Autodesk Fusion 360 part; units mm, degrees
sketch "Sketch1" plane through (0, 0, 0) normal (0, 0, 1) x (1, 0, 0)
  line L0 (-77.1661, 21.8494) -> (-77.196, -36.9915)
  line L1 (-55.1143, 21.8382) -> (-77.1661, 21.8494)
  line L2 (-55.1022, 45.5931) -> (-55.1143, 21.8382)
  line L3 (-35.4199, 45.5831) -> (-55.1022, 45.5931)
  line L4 (-35.4199, 55.6506) -> (-35.4199, 45.5831)
  line L5 (-16.3374, 55.6581) -> (-35.4199, 55.6506)
  line L6 (-16.3374, 65.0231) -> (-16.3374, 55.6581)
  line L7 (5.0551, 65.0106) -> (-16.3374, 65.0231)
  line L8 (5.0551, 55.3606) -> (5.0551, 65.0106)
  line L9 (24.2287, 55.413) -> (5.0551, 55.3606)
  line L10 (24.2287, 45.8698) -> (24.2287, 55.413)
  line L11 (43.6774, 45.8599) -> (24.2287, 45.8698)
  line L12 (43.6724, 36.0748) -> (43.6774, 45.8599)
  line L13 (72.4097, 36.0602) -> (43.6724, 36.0748)
  line L14 (72.377, -28.4302) -> (72.4097, 36.0602)
  line L15 (-18.082, -28.4553) -> (72.377, -28.4302)
  line L16 (-18.0799, -36.9775) -> (-18.082, -28.4553)
  line L17 (-77.196, -36.9915) -> (-18.0799, -36.9775)
  line L18 (-18.8374, 67.5106) -> (7.5551, 67.5106)
  line L19 (7.5551, 67.5106) -> (7.5551, 57.913)
  line L20 (7.5551, 57.913) -> (26.7287, 57.913)
  line L21 (26.7287, 57.913) -> (26.7287, 48.3599)
  line L22 (26.7287, 48.3599) -> (46.1774, 48.3599)
  line L23 (46.1774, 48.3599) -> (46.1774, 38.5602)
  line L24 (74.9097, 38.5602) -> (46.1774, 38.5602)
  line L25 (74.9097, 38.5602) -> (74.8744, -30.9302)
  line L26 (-15.5799, -30.9553) -> (-15.5799, -39.4775)
  line L27 (-15.5799, -30.9553) -> (74.8744, -30.9302)
  line L28 (-15.5799, -39.4775) -> (-79.696, -39.4775)
  line L29 (-79.696, -39.4775) -> (-79.6636, 24.3382)
  line L30 (-79.6636, 24.3382) -> (-57.6022, 24.3382)
  line L31 (-57.6022, 24.3382) -> (-57.6022, 48.0931)
  line L32 (-57.6022, 48.0931) -> (-37.9199, 48.0931)
  line L33 (-37.9199, 58.1581) -> (-37.9199, 48.0931)
  line L34 (-37.9199, 58.1581) -> (-18.8374, 58.1581)
  line L35 (-18.8374, 58.1581) -> (-18.8374, 67.5106)
  dimension "d1" = 2.5
  dimension "d2" = 2.5
  dimension "d4" = 2.5
  dimension "d5" = 2.5
  dimension "d6" = 2.5
  dimension "d7" = 2.5
  dimension "d8" = 2.5
  dimension "d9" = 2.5
  dimension "d11" = 2.5
  dimension "d12" = 2.5
  dimension "d13" = 2.5
  dimension "d14" = 2.5
  dimension "d16" = 2.5
  dimension "d17" = 2.5
  dimension "d18" = 2.5
  dimension "d19" = 2.5
  dimension "d20" = 2.5
  dimension "d21" = 2.5
  dimension "d22" = 2.5
extrude "Extrude1" add sketch "Sketch1" along normal blind 13
extrude "Extrude2" add sketch "Sketch1" along normal blind 3 contours L0 L1 L2 L3 L4 L5 L6 L7 L8 L9 L10 L11 L12 L13 L14 L15 L16 L17
sketch "Sketch4" plane through (0, 0, 13) normal (0, 0, 1) x (-1, 0, 0)
  line L0 (18.0799, 36.9775) -> (77.196, 36.9915)
  line L1 (77.196, 36.9915) -> (77.1661, -21.8494)
  line L2 (77.1661, -21.8494) -> (55.1143, -21.8382)
  line L3 (55.1143, -21.8382) -> (55.1022, -45.5931)
  line L4 (55.1022, -45.5931) -> (35.4199, -45.5831)
  line L5 (35.4199, -45.5831) -> (35.4199, -55.6506)
  line L6 (35.4199, -55.6506) -> (16.3374, -55.6581)
  line L7 (16.3374, -55.6581) -> (16.3374, -65.0231)
  line L8 (16.3374, -65.0231) -> (-5.0551, -65.0106)
  line L9 (-5.0551, -65.0106) -> (-5.0551, -55.3606)
  line L10 (-5.0551, -55.3606) -> (-24.2287, -55.413)
  line L11 (-24.2287, -55.413) -> (-24.2287, -45.8698)
  line L12 (-24.2287, -45.8698) -> (-43.6774, -45.8599)
  line L13 (-43.6774, -45.8599) -> (-43.6724, -36.0748)
  line L14 (-43.6724, -36.0748) -> (-72.4097, -36.0602)
  line L15 (-72.4097, -36.0602) -> (-72.377, 28.4302)
  line L16 (-72.377, 28.4302) -> (18.082, 28.4553)
  line L17 (18.082, 28.4553) -> (18.0799, 36.9775)
  line L18 (37.9199, -58.1581) -> (37.9199, -48.0931)
  line L19 (37.9199, -48.0931) -> (57.6022, -48.0931)
  line L20 (57.6022, -48.0931) -> (57.6022, -24.3382)
  line L21 (57.6022, -24.3382) -> (79.6636, -24.3382)
  line L22 (79.6636, -24.3382) -> (79.696, 39.4775)
  line L23 (79.696, 39.4775) -> (15.5799, 39.4775)
  line L24 (15.5799, 39.4775) -> (15.5799, 30.9553)
  line L25 (15.5799, 30.9553) -> (-74.8744, 30.9302)
  line L26 (-74.8744, 30.9302) -> (-74.9097, -38.5602)
  line L27 (-74.9097, -38.5602) -> (-46.1774, -38.5602)
  line L28 (-46.1774, -38.5602) -> (-46.1774, -48.3599)
  line L29 (-46.1774, -48.3599) -> (-26.7287, -48.3599)
  line L30 (-26.7287, -48.3599) -> (-26.7287, -57.913)
  line L31 (-26.7287, -57.913) -> (-7.5551, -57.913)
  line L32 (-7.5551, -57.913) -> (-7.5551, -67.5106)
  line L33 (-7.5551, -67.5106) -> (18.8374, -67.5106)
  line L34 (18.8374, -67.5106) -> (18.8374, -58.1581)
  line L35 (18.8374, -58.1581) -> (37.9199, -58.1581)
  line L36 (73.8436, -24.8) -> (60.8436, -24.8)
  line L37 (60.8436, -24.8) -> (60.8436, -21.5)
  line L38 (60.8436, -21.5) -> (73.8436, -21.5)
  line L39 (73.8436, -21.5) -> (73.8436, -24.8)
  dimension "d27" = 13
  dimension "d28" = 5.82
extrude "Extrude3" cut sketch "Sketch4" against normal blind 6 contours L2 L21 L37 L39
fillet "Fillet1" radius 1 18 edges at (-79.696, -39.4775, 6.5) (-15.5799, -39.4775, 6.5) (-15.5799, -30.9553, 6.5) (74.8744, -30.9302, 6.5) (74.9097, 38.5602, 6.5) (46.1774, 38.5602, 6.5) (26.7287, 48.3599, 6.5) (46.1774, 48.3599, 6.5) (26.7287, 57.913, 6.5) (7.5551, 67.5106, 6.5) (7.5551, 57.913, 6.5) (-57.6022, 48.0931, 6.5) (-57.6022, 24.3382, 6.5) (-79.6636, 24.3382, 6.5) (-37.9199, 48.0931, 6.5) (-37.9199, 58.1581, 6.5) (-18.8374, 58.1581, 6.5) (-18.8374, 67.5106, 6.5)
Check sheet for the modelled part. Datum: model origin and axes. Units: mm. A direction names the side the tool comes from. Coordinates: 2 decimals unless noted, no trailing zeros. Order: outer loops, then holes, each group sorted by start corner. A loop starts at its lowest first (then second) coordinate and runs counter-clockwise, first axis right, second up. Notation, with made-up numbers: (8.25, 42) -> (55.25, 42) arc R10 cw to (55.25, 49) -> close; hole circle Ø1 at (46.5, 3.25). An arc over 180 degrees is marked (long way). Write item = value, one per line. Start each with the question number.
1) Mould release check, pull along Y, two halves, no side actions. Record for faces 1 (the flat face through (-47, -39.478, 6)), 2 (the flat face through (-3, 3, 3)), 3 (the flat face through (7.555, 63, 6)), 4 (the flat face through (-6, 67.511, 6)): +Y half, -Y half, draft (parallel to the pull), parting line (faces both ways), or undercut.
2) Go/stop test with flat-tipped pins: P1, Ø1, axis at y = 8.5, z = 3, coming from the +X side; P2, Ø6.5, axis at x = -47, z = 9, coming from the +Y side; P3, Ø3, axis at y = 51.5, z = 7.5, coming from the -X side. Record where each tip stops, or that it passes through.
3) Cross-section at B-B (y = 31.5). Enter the section's corners in (x, z).
4) Cross-section at A-A (x = -67). Enter the section's corners in (y, z).
5) Access from +Z, -Z, +X, -X, +Y, -Y to the whole of each face (thin tool, end or side, straight path). Record for faces 5 (the flat face through (-14, -29, 13)), 6 (the flat face through (-48, 48.093, 6)), 7 (the flat face through (36, 48.36, 6)).
6) Material ranges on L1, parallel to Y at x = 62.5, z = 8.5; L2, parallel to Y at x = 23.5, z = 10.25; L3, parallel to X at y = 52.5, z = 4, recorded low to high.
Ans:
q1.face_1 = -Y half
q1.face_2 = undercut
q1.face_3 = draft
q1.face_4 = +Y half
q2.P1 = 74.89
q2.P2 = 48.09
q2.P3 = -37.92
q3.outline = (-57.6, 0) -> (74.91, 0) -> (74.91, 13) -> (72.41, 13) -> (72.41, 3) -> (-55.11, 3) -> (-55.11, 13) -> (-57.6, 13) -> close
q4.outline = (-39.48, 0) -> (24.34, 0) -> (24.34, 7) -> (21.84, 7) -> (21.84, 3) -> (-36.99, 3) -> (-36.99, 13) -> (-39.48, 13) -> close
q5.face_5 = +Z, +X, -X, +Y, -Y
q5.face_6 = +Z, -Z, -X, +Y
q5.face_7 = +Z, -Z, +X, +Y
q6.L1 = -30.93 to -28.43, 36.07 to 38.56
q6.L2 = -30.94 to -28.44, 55.41 to 57.91
q6.L3 = -37.92 to -35.42, 24.23 to 26.73
